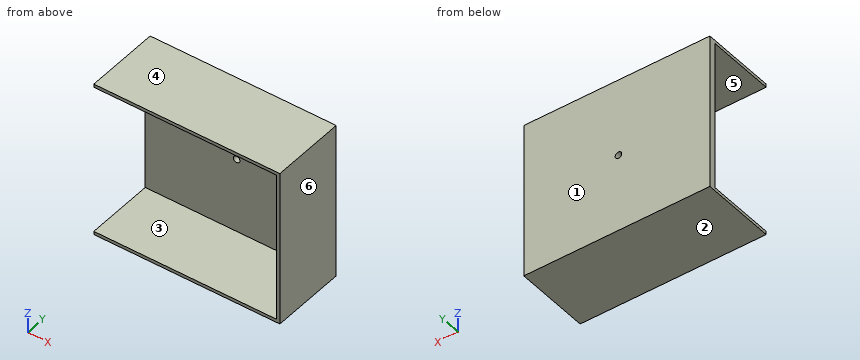
```python
from build123d import *

# Parameters (mm, degrees)
F0_W     = 71.12
F0_H     = 58.42
F0_H_2   = 1.27
F1_DEPTH = 29.21
F2_DEPTH = 29.211
F3_DEPTH = 2.54
F4_R     = 1.27
F5_DEPTH = 2.541


with BuildPart() as f1:
    # F0 (on Front) → F1 (new body)
    with BuildSketch(Plane.XZ):
        with Locations((35.56, 29.21)):
            Rectangle(F0_W, F0_H)
        with Locations((35.56, -0.635)):
            Rectangle(F0_W, F0_H_2)
        Polygon((71.12, 58.42), (71.12, 0), (71.12, -1.27), (72.39, -1.27), (72.39, 59.69), (71.12, 59.69), align=None)
        with Locations((35.56, 59.055)):
            Rectangle(F0_W, F0_H_2)
    extrude(amount=F1_DEPTH)

    # F0 (on Front) → F2 (cut, through all)
    with BuildSketch(Plane.XZ):
        with Locations((35.56, 29.21)):
            Rectangle(F0_W, F0_H)
    extrude(amount=F2_DEPTH, mode=Mode.SUBTRACT)

    # F0 (on Front) → F3 (join)
    with BuildSketch(Plane.XZ):
        with Locations((35.56, 29.21)):
            Rectangle(F0_W, F0_H)
    extrude(amount=F3_DEPTH)

    # F4 (on face) → F5 (cut, through all)
    with BuildSketch(Plane.XZ.offset(2.54)):
        with Locations((35.56, 29.21)):
            Circle(F4_R)
    extrude(amount=-F5_DEPTH, mode=Mode.SUBTRACT)


solid = f1.part
```
For this review, take the finished solid that the model builds, in its own axes (mm). Face numbers are marked on the shaded views. A direction names the side the tool comes from. Coordinates: 2 decimals unless noted, no trailing zeros. Write each loop counter-clockwise with the first axis right and the second up, starting at its lowest first coordinate (ties: lowest second). Pieces come first, ordered by that corner, then holes. Notation, with made-up numbers: (60.5, 15) - (81.5, 15) arc R23 ccw to (81.5, 25) - close; hole circle Ø11 at (56, -25). An arc over 180 degrees is marked (long way). Answer in a Markdown table with one row per item. Add a question column.
Q1. Draft analysis for pull direction Z (two halves, no side actions). For the marked faces 1, 2, 3 and 4, state which applies: +Z half, -Z half, draft (parallel to the pull), parting line (faces both ways), or undercut.
Q2. For P1, Ø17.5, axis at x = 50, z = 34.5, coming from the -Y side, flat-tipped, find the tip position at first contact; note if it passes through.
Q3. We need section B-B, the plane z = 29.21. State the section outline as (x, y) points, and give its area (3 significant figures).
Q4. We need section D-D, the plane y = -14.5. State the section outline as (x, z) points, and give its area (3 significant figures).
Q5. We need section C-C, the plane x = 48. State the section outline as (y, z) points, and give its area (3 significant figures).
Q6. Tool access review of the marked faces 5 and 6: name each direction out of +Z, -Z, +X, -X, +Y, -Y from which nothing blocks a thin tool from reaching the whole face with its end or side.
Q7. For probe 1 along Z at (x, y) = (60.5, -16.25); probe 2 along Z at (x, y) = (35.56, -1.65); probe 3 along Y at (x, z) = (56, 21), list the stretches that pass through material, from the lowest coordinate up.
Q8. We need section A-A, the plane x = 35.56. State the section outline as (y, z) points, and give its area (3 significant figures).
Answer list:
| question | item | result |
|---|---|---|
| 1 | face 1 | draft |
| 1 | face 2 | -Z half |
| 1 | face 3 | undercut |
| 1 | face 4 | +Z half |
| 2 | P1 | stops at y = -2.54 |
| 3 | outline | (0, -2.54) - (34.29, -2.54) - (34.29, 0) - (0, 0) - close; (36.83, -2.54) - (71.12, -2.54) - (71.12, -29.21) - (72.39, -29.21) - (72.39, 0) - (36.83, 0) - close |
| 3 | area | 211 mm2 |
| 4 | outline | (0, -1.27) - (72.39, -1.27) - (72.39, 59.69) - (0, 59.69) - (0, 58.42) - (71.12, 58.42) - (71.12, 0) - (0, 0) - close |
| 4 | area | 258 mm2 |
| 5 | outline | (-29.21, -1.27) - (0, -1.27) - (0, 59.69) - (-29.21, 59.69) - (-29.21, 58.42) - (-2.54, 58.42) - (-2.54, 0) - (-29.21, 0) - close |
| 5 | area | 223 mm2 |
| 6 | face 5 | -X, -Y |
| 6 | face 6 | +Z, -Z, +X, +Y, -Y |
| 7 | probe 1 | z = -1.27 to 0, 58.42 to 59.69 |
| 7 | probe 2 | z = -1.27 to 27.94, 30.48 to 59.69 |
| 7 | probe 3 | y = -2.54 to 0 |
| 8 | outline | (-29.21, -1.27) - (0, -1.27) - (0, 27.94) - (-2.54, 27.94) - (-2.54, 0) - (-29.21, 0) - close; (-29.21, 58.42) - (-2.54, 58.42) - (-2.54, 30.48) - (0, 30.48) - (0, 59.69) - (-29.21, 59.69) - close |
| 8 | area | 216 mm2 |
